```python
from build123d import *

# Parameters (mm, degrees)
SKETCH1_W                 = 139.7
SKETCH1_H                 = 139.7
BOSS_EXTRUDE1_DEPTH       = 3.175
SKETCH13_W                = 25.4
SKETCH13_H                = 3.175
CUT_EXTRUDE6_DEPTH        = 6.35
LPATTERN7_COUNT           = 2
LPATTERN7_PITCH           = 123.825
SKETCH14_W                = 3.175
SKETCH14_H                = 25.4
CUT_EXTRUDE7_DEPTH        = 6.35
F_8_CLEARANCE_HOLE1_D     = 4.4958
F_8_CLEARANCE_HOLE1_DEPTH = 10.16
F_8_CLEARANCE_HOLE1_TIP   = 1.350674586
SKETCH18_R                = 14.2875
CUT_EXTRUDE9_DEPTH        = 7.62
FILLET6_R                 = 12.7
CUT_EXTRUDE17_DEPTH       = 7.62
CIRPATTERN1_COUNT         = 4


with BuildPart() as part:
    # Sketch1 → Boss-Extrude1 (new body)
    with BuildSketch(Plane(origin=(0, 0, 0), x_dir=(1, 0, 0), z_dir=(0, 1, 0))):
        with Locations((69.85, 69.85)):
            Rectangle(SKETCH1_W, SKETCH1_H)
    extrude(amount=BOSS_EXTRUDE1_DEPTH)

    # Sketch13 → Cut-Extrude6 (cut)
    with BuildSketch(Plane(origin=(0, 3.175, 0), x_dir=(1, 0, 0), z_dir=(0, 1, 0))):
        with Locations((44.45, 7.9375)):
            Rectangle(SKETCH13_W, SKETCH13_H)
        with Locations((95.25, 7.9375)):
            Rectangle(SKETCH13_W, SKETCH13_H)
    cut_extrude6 = extrude(amount=-CUT_EXTRUDE6_DEPTH, mode=Mode.SUBTRACT)

    # LPattern7: Cut-Extrude6 ×2
    with Locations(*[(0, 0, -i * LPATTERN7_PITCH) for i in range(1, LPATTERN7_COUNT)]):
        add(cut_extrude6, mode=Mode.SUBTRACT)

    # Sketch14 → Cut-Extrude7 (cut)
    with BuildSketch(Plane(origin=(0, 3.175, 0), x_dir=(1, 0, 0), z_dir=(0, 1, 0))):
        with Locations((7.9375, 44.45)):
            Rectangle(SKETCH14_W, SKETCH14_H)
        with Locations((131.7625, 44.45)):
            Rectangle(SKETCH14_W, SKETCH14_H)
        with Locations((131.7625, 95.25)):
            Rectangle(SKETCH14_W, SKETCH14_H)
        with Locations((7.9375, 95.25)):
            Rectangle(SKETCH14_W, SKETCH14_H)
    extrude(amount=-CUT_EXTRUDE7_DEPTH, mode=Mode.SUBTRACT)

    # #8 Clearance Hole1
    with Locations(Plane(origin=(0, 3.175, 0), x_dir=(1, 0, 0), z_dir=(0, 1, 0))):
        with Locations((7.9375, 69.85), (131.826, 69.85)):
            Hole(F_8_CLEARANCE_HOLE1_D / 2, depth=F_8_CLEARANCE_HOLE1_DEPTH)
            with Locations((0, 0, -(F_8_CLEARANCE_HOLE1_DEPTH + F_8_CLEARANCE_HOLE1_TIP / 2))):  # 118° drill point
                Cone(0, F_8_CLEARANCE_HOLE1_D / 2, F_8_CLEARANCE_HOLE1_TIP, mode=Mode.SUBTRACT)

    # Sketch18 → Cut-Extrude9 (cut)
    with BuildSketch(Plane(origin=(0, 3.175, 0), x_dir=(1, 0, 0), z_dir=(0, 1, 0))):
        with Locations(Location((69.85, 69.85, 0), (0, 0, 270))):
            Circle(SKETCH18_R)
    extrude(amount=-CUT_EXTRUDE9_DEPTH, mode=Mode.SUBTRACT)

    # Fillet6
    fillet6_edges = [part.edges().sort_by_distance(p)[0] for p in [
        (0, 1.5875, -139.7),
        (139.7, 1.5875, -139.7),
        (139.7, 1.5875, 0),
        (0, 1.5875, 0),
    ]]
    fillet(fillet6_edges, radius=FILLET6_R)

    # Sketch26 → Cut-Extrude17 (cut)
    with BuildSketch(Plane(origin=(0, 3.175, 0), x_dir=(1, 0, 0), z_dir=(0, 1, 0))):
        with BuildLine():
            ThreePointArc((66.675, 114.186462139), (38.419103576, 101.280896424), (25.513537861, 73.025))
            Line((25.513537861, 73.025), (38.259148872, 73.025))
            ThreePointArc((38.259148872, 73.025), (47.399359697, 92.300640303), (66.675, 101.440851128))
            Line((66.675, 101.440851128), (66.675, 114.186462139))
        make_face()
        with BuildLine():
            ThreePointArc((25.513537861, 66.675), (38.419103576, 38.419103576), (66.675, 25.513537861))
            Line((66.675, 25.513537861), (66.675, 38.259148872))
            ThreePointArc((66.675, 38.259148872), (47.399359697, 47.399359697), (38.259148872, 66.675))
            Line((38.259148872, 66.675), (25.513537861, 66.675))
        make_face()
        with BuildLine():
            Line((73.025, 38.259148872), (73.025, 25.513537861))
            ThreePointArc((73.025, 25.513537861), (101.280896424, 38.419103576), (114.186462139, 66.675))
            Line((114.186462139, 66.675), (101.440851128, 66.675))
            ThreePointArc((101.440851128, 66.675), (92.300640303, 47.399359697), (73.025, 38.259148872))
        make_face()
        with BuildLine():
            Line((101.440851128, 73.025), (114.186462139, 73.025))
            ThreePointArc((114.186462139, 73.025), (101.280896424, 101.280896424), (73.025, 114.186462139))
            Line((73.025, 114.186462139), (73.025, 101.440851128))
            ThreePointArc((73.025, 101.440851128), (92.300640303, 92.300640303), (101.440851128, 73.025))
        make_face()
    extrude(amount=-CUT_EXTRUDE17_DEPTH, mode=Mode.SUBTRACT)

    # Sketch27 → #4 Clearance Hole1 (revolve, cut)
    with BuildSketch(Plane(origin=(69.85, 3.175, -107.95), x_dir=(0, 0, 1), z_dir=(1, 0, 0))):
        Polygon((0, 0), (0, 11.140574487), (1.63195, 10.16), (1.63195, 0), align=None)
    f_4_clearance_hole1 = revolve(axis=Axis((69.85, 9.525, -107.95), (0, -1, 0)), mode=Mode.SUBTRACT)

    # CirPattern1: #4 Clearance Hole1 ×4 about axis
    cirpattern1_axis = Axis((69.85, 0, -69.85), (0, 1, 0))
    for i in range(1, CIRPATTERN1_COUNT):
        add(f_4_clearance_hole1.rotate(cirpattern1_axis, i * 360 / CIRPATTERN1_COUNT), mode=Mode.SUBTRACT)


solid = part.part
```
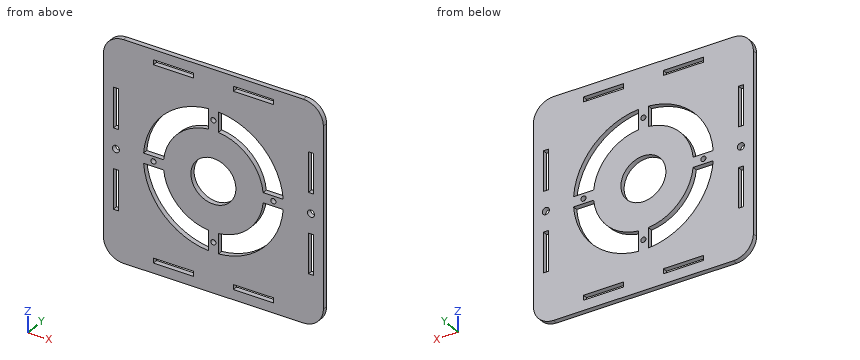
Can you work these out from the model? Positions are in its coordinate system, mm. Round coordinates to 2 decimals unless told otherwise and drop trailing zeros. Loops run counter-clockwise (first coordinate to the right, second up) from the corner with the lowest first, then second, coordinate; pieces in that order, holes last. Notation, with made-up numbers: (9, -22.5) -> (52, -22.5) arc R11 ccw to (52, -18.5) -> close; hole circle Ø4 at (17, 35). An arc over 180 degrees is marked (long way). One line per item, written item: value. Start each with the question number.
1. If we section it at B-B, the plane z = -76: Write out the boundary of the cut face in (x, y) (1 decimal).
2. If we section it at A-A, the plane x = 69.85: Write out the boundary of the cut face in (y, z) (1 decimal).
3. If we section it at C-C, the plane x = 95: Write out the boundary of the cut face in (y, z) (3 decimals).
4. For pin 1 (1.6 mm diameter, centred on y = 1, z = -8.5, fed in from +X); pin 2 (5 mm diameter, centred on x = 69.85, z = -107.95, fed in from -Y); pin 3 (1 mm diameter, centred on x = 7.5, y = 2, fed in from +Z), each with a flat end and sliding along its axis, tell me the tip position at first contact or that it passes through.
5. If I drill on probe 1 along X at (y, z) = (2.2, -30.5) (3 decimals); probe 2 along X at (y, z) = (0.9, -133); probe 3 along X at (y, z) = (2.8, -105) (3 decimals), over which ranges is the centre line in solid material (lowest first)?
6. If we section it at D-D, the plane y = 2.2: Give the number of separate pieces and of enclosed holes in the cut face, then the cut area to 3 significant figures.
Calculated:
1. outline: (0, 0) -> (25.8, 0) -> (25.8, 3.2) -> (0, 3.2) -> close; (38.7, 0) -> (57, 0) -> (57, 3.2) -> (38.7, 3.2) -> close; (82.7, 0) -> (101, 0) -> (101, 3.2) -> (82.7, 3.2) -> close; (113.9, 0) -> (139.7, 0) -> (139.7, 3.2) -> (113.9, 3.2) -> close
2. outline: (0, -139.7) -> (3.2, -139.7) -> (3.2, -109.6) -> (0, -109.6) -> close; (0, -106.3) -> (3.2, -106.3) -> (3.2, -84.1) -> (0, -84.1) -> close; (0, -55.6) -> (3.2, -55.6) -> (3.2, -33.4) -> (0, -33.4) -> close; (0, -30.1) -> (3.2, -30.1) -> (3.2, 0) -> (0, 0) -> close
3. outline: (0, -139.7) -> (3.175, -139.7) -> (3.175, -133.35) -> (0, -133.35) -> close; (0, -130.175) -> (3.175, -130.175) -> (3.175, -106.501) -> (0, -106.501) -> close; (0, -89.229) -> (3.175, -89.229) -> (3.175, -50.471) -> (0, -50.471) -> close; (0, -33.199) -> (3.175, -33.199) -> (3.175, -9.525) -> (0, -9.525) -> close; (0, -6.35) -> (3.175, -6.35) -> (3.175, 0) -> (0, 0) -> close
4. pin 1: stops at x = 139.24
4. pin 2: stops at y = 0
4. pin 3: stops at z = -0.9
5. probe 1: x = 0 to 49.177, 66.675 to 68.801, 70.899 to 73.025, 90.523 to 139.7
5. probe 2: x = 1.51 to 31.75, 57.15 to 82.55, 107.95 to 138.19
5. probe 3: x = 0 to 6.35, 9.525 to 42.642, 66.675 to 73.025, 97.058 to 130.175, 133.35 to 139.7
6. separate pieces: 1
6. enclosed holes: 19
6. area: 15,300 mm²
